Could you check a few things on this model? Use its own coordinates, in mm. A direction names the side the tool comes from. Give positions to 0.01 mm unless a question says otherwise; leave off trailing zeros.
from build123d import *

# Parameters (mm, degrees)
BOSS_EXTRUDE1_DEPTH             = 330
M6X1_0_TAPPED_HOLE2_D           = 5
M6X1_0_TAPPED_HOLE2_DEPTH       = 28.497848452
M6X1_0_TAPPED_HOLE2_CSINK_D     = 6.05
M6X1_0_TAPPED_HOLE2_CSINK_ANGLE = 90
M6X1_0_TAPPED_HOLE2_TIP         = 1.502151548


with BuildPart() as part:
    # Sketch1 → Boss-Extrude1 (new body)
    with BuildSketch(Plane.XY):
        with BuildLine():
            Line((-9.5, 10), (-3.486470896, 10))
            ThreePointArc((-3.486470896, 10), (-3.373276191, 9.726723809), (-3.1, 9.613529104))
            Line((-3.1, 9.613529104), (-3.1, 8.7))
            Line((-3.1, 8.7), (-3.6, 8.2))
            Line((-3.6, 8.2), (-5, 8.2))
            Line((-5, 8.2), (-5.5, 7.7))
            Line((-5.5, 7.7), (-5.5, 6.560660172))
            Line((-5.5, 6.560660172), (-2.839339828, 3.9))
            Line((-2.839339828, 3.9), (0, 3.9))
            Line((0, 3.9), (2.839339828, 3.9))
            Line((2.839339828, 3.9), (5.5, 6.560660172))
            Line((5.5, 6.560660172), (5.5, 7.7))
            Line((5.5, 7.7), (5, 8.2))
            Line((5, 8.2), (3.1, 8.2))
            Line((3.1, 8.2), (3.1, 9.613529104))
            ThreePointArc((3.1, 9.613529104), (3.373276191, 9.726723809), (3.486470896, 10))
            Line((3.486470896, 10), (9.5, 10))
            Line((9.5, 10), (10, 9.5))
            Line((10, 9.5), (10, 3.486470896))
            ThreePointArc((10, 3.486470896), (9.726723809, 3.373276191), (9.613529104, 3.1))
            Line((9.613529104, 3.1), (8.7, 3.1))
            Line((8.7, 3.1), (8.2, 3.6))
            Line((8.2, 3.6), (8.2, 5))
            Line((8.2, 5), (7.7, 5.5))
            Line((7.7, 5.5), (6.560660172, 5.5))
            Line((6.560660172, 5.5), (3.9, 2.839339828))
            Line((3.9, 2.839339828), (3.9, 0))
            Line((3.9, 0), (3.9, -2.839339828))
            Line((3.9, -2.839339828), (6.560660172, -5.5))
            Line((6.560660172, -5.5), (7.7, -5.5))
            Line((7.7, -5.5), (8.2, -5))
            Line((8.2, -5), (8.2, -3.1))
            Line((8.2, -3.1), (9.613529104, -3.1))
            ThreePointArc((9.613529104, -3.1), (9.726723809, -3.373276191), (10, -3.486470896))
            Line((10, -3.486470896), (10, -9.5))
            Line((10, -9.5), (9.5, -10))
            Line((9.5, -10), (3.486470896, -10))
            ThreePointArc((3.486470896, -10), (3.373276191, -9.726723809), (3.1, -9.613529104))
            Line((3.1, -9.613529104), (3.1, -8.7))
            Line((3.1, -8.7), (3.6, -8.2))
            Line((3.6, -8.2), (5, -8.2))
            Line((5, -8.2), (5.5, -7.7))
            Line((5.5, -7.7), (5.5, -6.560660172))
            Line((5.5, -6.560660172), (2.839339828, -3.9))
            Line((2.839339828, -3.9), (0, -3.9))
            Line((0, -3.9), (-2.839339828, -3.9))
            Line((-2.839339828, -3.9), (-5.5, -6.560660172))
            Line((-5.5, -6.560660172), (-5.5, -7.7))
            Line((-5.5, -7.7), (-5, -8.2))
            Line((-5, -8.2), (-3.1, -8.2))
            Line((-3.1, -8.2), (-3.1, -9.613529104))
            ThreePointArc((-3.1, -9.613529104), (-3.373276191, -9.726723809), (-3.486470896, -10))
            Line((-3.486470896, -10), (-9.5, -10))
            Line((-9.5, -10), (-10, -9.5))
            Line((-10, -9.5), (-10, -3.486470896))
            ThreePointArc((-10, -3.486470896), (-9.726723809, -3.373276191), (-9.613529104, -3.1))
            Line((-9.613529104, -3.1), (-8.7, -3.1))
            Line((-8.7, -3.1), (-8.2, -3.6))
            Line((-8.2, -3.6), (-8.2, -5))
            Line((-8.2, -5), (-7.7, -5.5))
            Line((-7.7, -5.5), (-6.560660172, -5.5))
            Line((-6.560660172, -5.5), (-3.9, -2.839339828))
            Line((-3.9, -2.839339828), (-3.9, 0))
            Line((-3.9, 0), (-3.9, 2.839339828))
            Line((-3.9, 2.839339828), (-6.560660172, 5.5))
            Line((-6.560660172, 5.5), (-7.7, 5.5))
            Line((-7.7, 5.5), (-8.2, 5))
            Line((-8.2, 5), (-8.2, 3.1))
            Line((-8.2, 3.1), (-9.613529104, 3.1))
            ThreePointArc((-9.613529104, 3.1), (-9.726723809, 3.373276191), (-10, 3.486470896))
            Line((-10, 3.486470896), (-10, 9.5))
            Line((-10, 9.5), (-9.5, 10))
        make_face()
    extrude(amount=BOSS_EXTRUDE1_DEPTH)

    # Sketch2 → M6x1.0 Tapped Hole1 (revolve, cut)
    with BuildSketch(Plane(origin=(0, 0, 330), x_dir=(0, -1, 0), z_dir=(1, 0, 0))):
        Polygon((0, 0), (0, 30), (2.5, 28.497848452), (2.5, 0.525), (3.025, 0), align=None)
    revolve(axis=Axis((0, 0, 336.35), (0, 0, -1)), mode=Mode.SUBTRACT)

    # M6x1.0 Tapped Hole2
    with Locations(Plane(origin=(0, 0, 0), x_dir=(-1, 0, 0), z_dir=(0, 0, -1))):
        with Locations((0, 0)):
            CounterSinkHole(M6X1_0_TAPPED_HOLE2_D / 2, M6X1_0_TAPPED_HOLE2_CSINK_D / 2, depth=M6X1_0_TAPPED_HOLE2_DEPTH, counter_sink_angle=M6X1_0_TAPPED_HOLE2_CSINK_ANGLE)
            with Locations((0, 0, -(M6X1_0_TAPPED_HOLE2_DEPTH + M6X1_0_TAPPED_HOLE2_TIP / 2))):  # 118° drill point
                Cone(0, M6X1_0_TAPPED_HOLE2_D / 2, M6X1_0_TAPPED_HOLE2_TIP, mode=Mode.SUBTRACT)


solid = part.part
Item 1: For faces 5 (the flat face through (10, 7, 163)), 6 (the flat face through (0, 3.9, 163)), 7 (the flat face through (-7, 10, 163)), 8 (the cylindrical face through (-0.54, -2.44, 14.71)), 9 (the flat face through (3.9, 0, 163)), which set-ups out of +Z, -Z, +X, -X, +Y, -Y let a thin tool reach every point of the face, with its end or its side?
Findings:
face 5: +Z, -Z, +X, +Y, -Y
face 6: +Z, -Z, +Y
face 7: +Z, -Z, +X, -X, +Y
face 8: -Z
face 9: +Z, -Z, +X
Item 2: For pin 1 (4 mm diameter, centred on x = 0, y = 0, fed in from +Z); pin 2 (3 mm diameter, centred on x = -0.5, z = 138.5, fed in from -Y); pin 3 (1.7 mm diameter, centred on y = 0, z = 242.5, fed in from -X), each with a flat end and sliding along its axis, tell me the tip position at first contact or that it passes through.
Findings:
pin 1: stops at z = 301.2
pin 2: stops at y = -3.9
pin 3: stops at x = -3.9
Item 3: We'd pull the mould along X, two halves only. Please class faces 1 (the cylindrical face through (2.44, 0.54, 315.68)), 2 (the flat face through (10, -6, 163)), 3 (the flat face through (2.4, 2.4, 0)), 4 (the flat face through (-10, 6, 163)): +X half, -X half, draft (parallel to the pull), parting line (faces both ways), or undercut.
Findings:
face 1: undercut
face 2: +X half
face 3: draft
face 4: -X half
Item 4: Please list where these lines run through material, in increasing order: line 1 along Y through (x, z) = (0, 21.5); line 2 along X through (y, z) = (-7.75, 112).
Findings:
line 1: y = -3.9 to -2.5, 2.5 to 3.9
line 2: x = -10 to -5.45, 5.45 to 10
